```python
from build123d import *

# Parameters (mm, degrees)
F0_R     = 112.5
F1_DEPTH = 14.9
F2_R     = 80
F3_DEPTH = 16.1
F4_SIZE  = 2
F5_R     = 74.5
F6_DEPTH = 31.001
F8_D     = 14


with BuildPart() as f1:
    # F0 (on Right) → F1 (new body)
    with BuildSketch(Plane.YZ):
        Circle(F0_R)
    extrude(amount=F1_DEPTH)

    # F2 (on face) → F3 (join)
    with BuildSketch(Plane(origin=(0, 0, 0), x_dir=(0, -1, 0), z_dir=(-1, 0, 0))):
        Circle(F2_R)
    extrude(amount=F3_DEPTH)

    # F4
    f4_edges = [f1.edges().sort_by_distance(p)[0] for p in [
        (-16.1, 80, 0),
        (14.9, -112.5, 0),
    ]]
    chamfer(f4_edges, length=F4_SIZE)

    # F5 (on face) → F6 (cut, through all)
    with BuildSketch(Plane(origin=(-16.1, 0, 0), x_dir=(0, -1, 0), z_dir=(-1, 0, 0))):
        Circle(F5_R)
    extrude(amount=-F6_DEPTH, mode=Mode.SUBTRACT)

    # F8 (through all)
    with Locations(Plane.YZ.offset(14.9)):
        with Locations((0, -93), (-93, 0), (0, 93), (93, 0)):
            Hole(F8_D / 2)


solid = f1.part
```
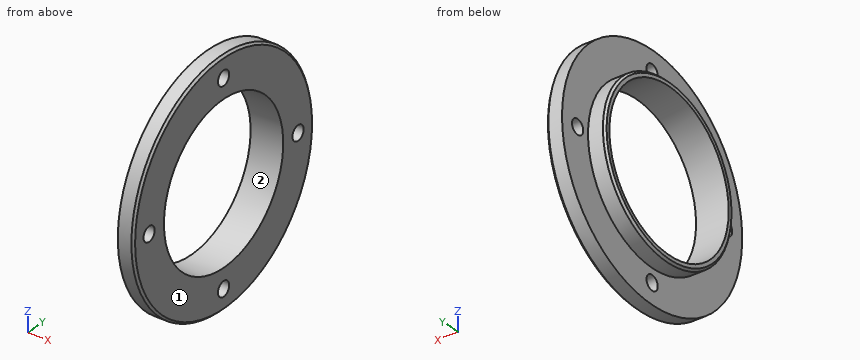
The listing builds one solid part. Answer for the finished solid, in the listing's coordinates (mm). Face numbers are marked on the shaded views. Give positions to 0.01 mm unless a question says otherwise; leave off trailing zeros. Order: outer loops, then holes, each group sorted by start corner. A loop starts at its lowest first (then second) coordinate and runs counter-clockwise, first axis right, second up. Notation, with made-up numbers: (-8.5, 69.25) -> (2.5, 69.25) arc R12 cw to (2.5, 86.25) -> close; hole circle Ø5 at (85, 27). An arc over 180 degrees is marked (long way). Write each question's results on one line, items separated by ' | '.
Q1. Determine the mould class of the marked faces 1 and 2 for opening direction Y: pulls with the +Y half, pulls with the -Y half, needs draft (parallel to the pull), parting line crosses it, or undercut.
Checked values:
face 1: needs draft | face 2: undercut
Q2. The part is cut by section A-A, the plane y = 0. Give the vertices of the cut face in (x, z), and give its area (3 significant figures).
Checked values:
outline: (-16.1, -78) -> (-14.1, -80) -> (0, -80) -> (0, -86) -> (14.9, -86) -> (14.9, -74.5) -> (-16.1, -74.5) -> close; (-16.1, 74.5) -> (14.9, 74.5) -> (14.9, 86) -> (0, 86) -> (0, 80) -> (-14.1, 80) -> (-16.1, 78) -> close; (0, -112.5) -> (12.9, -112.5) -> (14.9, -110.5) -> (14.9, -100) -> (0, -100) -> close; (0, 100) -> (14.9, 100) -> (14.9, 110.5) -> (12.9, 112.5) -> (0, 112.5) -> close | area: 884 mm^2
Q3. The part is cut by section D-D, the plane x = -7. Give the vertices of the cut face in (y, z), and give its area (3 significant figures).
Checked values:
outline: circle Ø160 at (0, 0); hole circle Ø149 at (0, 0) | area: 2,670 mm^2
Q4. Each of these flat-tipped pins is pushed along its axis until it touches: P1, Ø3, axis at x = 2.5, y = 78, coming from the +Z side; P2, Ø22.5, axis at y = -93, z = 0, coming from the -X side; P3, Ø10, axis at x = -1, z = 21.5, coming from the +Y side. Where does it stop, or does it pass through?
Checked values:
P1: stops at z = 82.49 | P2: stops at x = 0 | P3: stops at y = 111.27
Q5. Straight lines are drawn through the part: probe 1 along Z at (x, y) = (7.5, 0); probe 2 along Y at (x, z) = (-1, 1); probe 3 along X at (y, z) = (91.5, 8). For each, find the intervals that lie inside material, in ascending order. Write a range as from..to.
Checked values:
probe 1: z = -112.5..-100, -86..-74.5, 74.5..86, 100..112.5 | probe 2: y = -79.99..-74.49, 74.49..79.99 | probe 3: x = 0..14.9
Q6. The part is cut by section C-C, the plane x = 5.5. Give the vertices of the cut face in (y, z).
Checked values:
outline: circle Ø225 at (0, 0); hole circle Ø14 at (-93, 0); hole circle Ø149 at (0, 0); hole circle Ø14 at (0, -93); hole circle Ø14 at (0, 93); hole circle Ø14 at (93, 0)
